The model under review builds one solid part; all positions refer to its coordinate system, in mm. A direction names the side the tool comes from. Round coordinates to 2 decimals unless told otherwise and drop trailing zeros. Order: outer loops, then holes, each group sorted by start corner. A loop starts at its lowest first (then second) coordinate and runs counter-clockwise, first axis right, second up. Notation, with made-up numbers: M 73.5,-1 L 112.5,-1 A19 cw 112.5,8 Z; hole C 35.5,-12.75 d1. An arc over 180 degrees is marked long. Use a Markdown table: item, result. Add a question column.
1. For faces 4 (the flat face through (-6.245, 6.294, 1.275)), 5 (the flat face through (-6.2, 6.7, 2.07)), list the 3-axis set-ups (+Z, -Z, +X, -X, +Y, -Y) from which the entire face can be reached by the end or side of a thin tool; tool diameter is ignored.
2. Consider section C-C on x = -5.5. State the section outline as (y, z) points, then the cut area to 3 significant figures.
3. Consider section B-B on x = -14.75. State the section outline as (y, z) points, then the cut area to 3 significant figures.
4. Consider section D-D on y = 7.5. State the section outline as (x, z) points.
5. The part is to be moulded in two halves that separate along Z. For faces 1 (the cylindrical face through (-15.416, 6.648, 1.248)), 2 (the flat face through (-15.926, 7, 1)), 3 (the flat face through (-6.3, 6.7, 0.458)), say which applies: +Z half, -Z half, draft (parallel to the pull), parting line (faces both ways), or undercut.
6. To check wall thickness, follow probe 1 along Z at (x, y) = (-9.75, 6.3); probe 2 along Z at (x, y) = (-14.25, 6.6); probe 3 along X at (y, z) = (7.1, 1.95). State the ranges of each line that lie inside material, in increasing order.
7. Consider section A-A on z = 1.55. State the section outline as (x, y) points.
8. Insertion check: P1, Ø1, axis at x = -9.5, z = 2, coming from the -Y side. The pin has a flat end and moves straight along its axis. Give the tip position at first contact, or say it passes through.
Autodesk Inventor part; units mm, degrees
ref_plane "YZ Plane" through (0, 0, 0) normal (1, 0, 0) x (0, 1, 0)
ref_plane "XZ Plane" through (0, 0, 0) normal (0, 1, 0) x (-1, 0, 0)
ref_plane "XY Plane" through (0, 0, 0) normal (0, 0, 1) x (1, 0, 0)
sketch "Sketch1" plane through (0, 0, 0) normal (0, 0, 1) x (1, 0, 0)
  line L0 (-15.9265, 7.9959) -> (-1.5469, 7.9959)
  line L1 (-15.9265, 5.1636) -> (-15.9265, 7.9959)
  line L2 (-15.9265, 5.1636) -> (-1.5469, 7.9959)
  point P0 (0, 0)
extrude "Extrusion1" add sketch "Sketch1" along normal blind 2.54
sketch "Sketch2" plane through (-1.5469, 7.9959, 0) normal (0.1932565, -0.9811483, 0) x (0.9811483, 0.1932565, 0)
  line L0 (-1.1823, 2.0698) -> (-8.5899, 2.0698)
  line L1 (-8.5899, 2.0698) -> (-8.5899, 0.4575)
  line L2 (-8.5899, 0.4575) -> (-1.1823, 0.4575)
  line L3 (-1.1823, 0.4575) -> (-1.1823, 2.0698)
  point P0 (-0.0275, 0)
extrude "Extrusion2" add sketch "Sketch2" along normal blind 0.762
sketch "Sketch3" plane through (-15.9265, 7.9959, 0) normal (0, 1, 0) x (1, 0, 0)
  circle A0 centre (1.3508, -1.2855) radius 0.8416
  point P0 (15.9265, 0)
extrude "Extrusion3" cut sketch "Sketch3" against normal blind 12.7
properties part number "GRIPPER2"
Answer block:
| question | item | result |
|---|---|---|
| 1 | face 4 | +Z, -Z, +X, -Y |
| 1 | face 5 | +Z, +X, -Y |
| 2 | outline | M 6.44,0.46 L 7.22,0.46 L 7.22,0 L 8,0 L 8,2.54 L 7.22,2.54 L 7.22,2.07 L 6.44,2.07 Z |
| 2 | area | 3.23 mm^2 |
| 3 | outline | M 5.4,0 L 8,0 L 8,0.46 L 5.4,0.46 Z; M 5.4,2.11 L 8,2.11 L 8,2.54 L 5.4,2.54 Z |
| 3 | area | 2.32 mm^2 |
| 4 | outline | M -15.93,0 L -4.06,0 L -4.06,0.46 L -2.65,0.46 L -2.65,2.07 L -4.06,2.07 L -4.06,2.54 L -15.93,2.54 Z; hole C -14.58,1.29 d1.68 |
| 5 | face 1 | undercut |
| 5 | face 2 | draft |
| 5 | face 3 | -Z half |
| 6 | probe 1 | 0.46 to 2.07 |
| 6 | probe 2 | 0 to 0.51, 2.06 to 2.54 |
| 6 | probe 3 | -15.93 to -15.09, -14.06 to -2.58 |
| 7 | outline | M -15.93,5.16 L -15.37,5.27 L -15.37,8 L -15.93,8 Z; M -13.78,5.59 L -9.97,6.34 L -9.83,5.59 L -2.56,7.02 L -2.71,7.77 L -1.55,8 L -13.78,8 Z |
| 8 | P1 | y = 5.59 |
